Input: dimensioned drawing with shaded views. Units: mm. Origin: part minimum x, y, z. A direction names the side the tool comes from. Give positions to 0.01 mm unless a question says otherwise; leave off trailing zeros. Order: outer loops, then holes, each group sorted by start corner. A loop starts at its lowest first (then second) coordinate and runs counter-clockwise, first axis right, second up. Notation, with made-up numbers: (30, -25.5) - (35, -25.5) arc R26 cw to (35, 11.5) - close; hole circle Ø3 at (15.5, -14). An arc over 180 degrees is marked (long way). Answer as CSV lines item,"result".
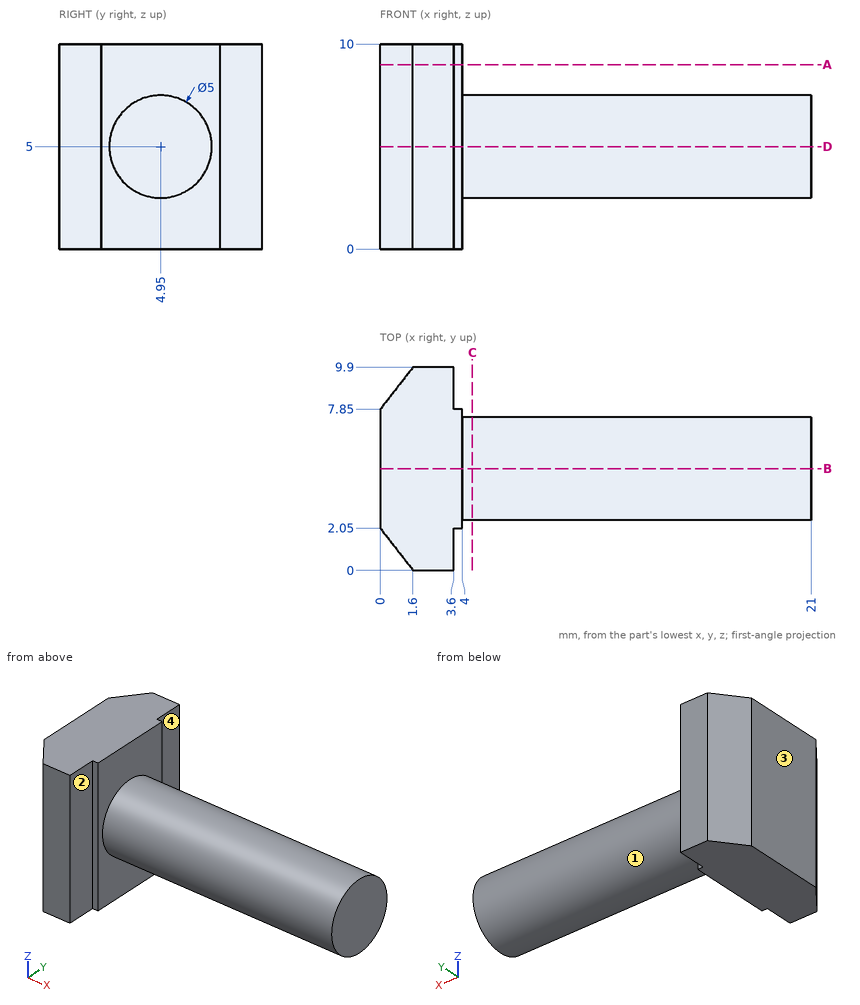
(1) Ray query, line 1 (X direction, y = 7.75, z = 9.75); line 2 (Y direction, x = 3.75, z = 1); line 3 (Y direction, x = 1.5, z = 8). Return the intervals inside material, ascending. Write a range as from..to.
Completed:
line 1,"0..4"
line 2,"2.05..7.85"
line 3,"0.13..9.77"
(2) Cut plane A-A (z = 9). Return loops of the section in (x, y).
Completed:
outline,"(0, 2.05) - (1.6, 0) - (3.6, 0) - (3.6, 2.05) - (4, 2.05) - (4, 7.85) - (3.6, 7.85) - (3.6, 9.9) - (1.6, 9.9) - (0, 7.85) - close"
(3) Cut plane B-B (y = 4.95). Return loops of the section in (x, z), then the cut area to 3 significant figures.
Completed:
outline,"(0, 0) - (4, 0) - (4, 2.5) - (21, 2.5) - (21, 7.5) - (4, 7.5) - (4, 10) - (0, 10) - close"
area,"125 mm²"
(4) Cut plane C-C (x = 4.5). Return loops of the section in (y, z), then the cut area to 3 significant figures.
Completed:
outline,"circle Ø5 at (4.95, 5)"
area,"19.6 mm²"
(5) Cut plane D-D (z = 5). Return loops of the section in (x, y), then the cut area to 3 significant figures.
Completed:
outline,"(0, 2.05) - (1.6, 0) - (3.6, 0) - (3.6, 2.05) - (4, 2.05) - (4, 2.45) - (21, 2.45) - (21, 7.45) - (4, 7.45) - (4, 7.85) - (3.6, 7.85) - (3.6, 9.9) - (1.6, 9.9) - (0, 7.85) - close"
area,"120 mm²"
(6) Access query for the marked faces 1, 2, 3 and 4. Directions: +Z, -Z, +X, -X, +Y, -Y. A direction counts if a zero-diameter tool reaches every point of the face in a straight line with its end or side. Return the directions, or none.
Completed:
face 1,"+X"
face 2,"+Z, -Z, +X, -Y"
face 3,"+Z, -Z, -X, +Y, -Y"
face 4,"+Z, -Z, +X, +Y"
(7) Contact query for flat-ended pins moving along their axis: pin 1 (1.6 mm diameter, centred on y = 0.5, z = 5, fed in from +X); pin 2 (5 mm diameter, centred on x = 18.5, z = 2, fed in from +Y); pin 3 (2 mm diameter, centred on x = 18, z = 2, fed in from -Y). Output: stop coordinate, or through.
Completed:
pin 1,"x = 3.6"
pin 2,"y = 7.4"
pin 3,"y = 3.45"
